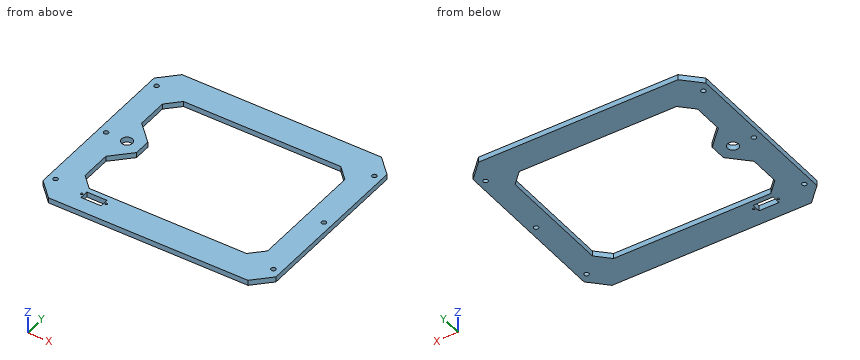
from build123d import *

# Parameters (mm, degrees)
SKETCH1_W           = 278
SKETCH1_H           = 238
BOSS_EXTRUDE1_DEPTH = 6.35
CHAMFER1_SIZE       = 20
SKETCH4_R           = 2.75
CUT_EXTRUDE2_DEPTH  = 76.2
SKETCH5_R           = 6.5
CUT_EXTRUDE3_DEPTH  = 10
SKETCH7_R           = 1.25
SKETCH7_W           = 24
SKETCH7_H           = 10.5
CUT_EXTRUDE4_DEPTH  = 7.35


with BuildPart() as part:
    # Sketch1 → Boss-Extrude1 (new body)
    with BuildSketch(Plane.XY):
        Rectangle(SKETCH1_W, SKETCH1_H)
    extrude(amount=BOSS_EXTRUDE1_DEPTH)

    # Chamfer1
    chamfer1_edges = [part.edges().sort_by_distance(p)[0] for p in [
        (-139, 119, 3.175),
        (139, 119, 3.175),
        (139, -119, 3.175),
        (-139, -119, 3.175),
    ]]
    chamfer(chamfer1_edges, length=CHAMFER1_SIZE)

    # Sketch4 → Cut-Extrude2 (cut)
    with BuildSketch(Plane.XY.offset(6.35)):
        with Locations((-130, 90)):
            Circle(SKETCH4_R)
        with Locations((-130, -90)):
            Circle(SKETCH4_R)
        with Locations((-130, 0)):
            Circle(SKETCH4_R)
        with Locations((130, -90)):
            Circle(SKETCH4_R)
        with Locations((130, 0)):
            Circle(SKETCH4_R)
        with Locations((130, 90)):
            Circle(SKETCH4_R)
    extrude(amount=-CUT_EXTRUDE2_DEPTH, mode=Mode.SUBTRACT)

    # Sketch5 → Cut-Extrude3 (cut)
    with BuildSketch(Plane.XY.offset(6.35)):
        with Locations((-105, 0)):
            Circle(SKETCH5_R)
        Polygon((93.875716073, -84), (-93.875716073, -84), (-108.875716073, -69), (-108.875716073, -32), (-86.875716073, -10), (-86.875716073, 10), (-108.875716073, 32), (-108.875716073, 69), (-93.875716073, 84), (93.875716073, 84), (108.875716073, 69), (108.875716073, -69), align=None)
    extrude(amount=-CUT_EXTRUDE3_DEPTH, mode=Mode.SUBTRACT)

    # Sketch7 → Cut-Extrude4 (cut, through all)
    with BuildSketch(Plane.XY.offset(6.35)):
        with Locations((-66.115841415, -95.342057099)):
            Circle(SKETCH7_R)
        with Locations((-95.115841415, -95.342057099)):
            Circle(SKETCH7_R)
        with Locations((-80.615841415, -95.342057099)):
            Rectangle(SKETCH7_W, SKETCH7_H)
    extrude(amount=-CUT_EXTRUDE4_DEPTH, mode=Mode.SUBTRACT)


solid = part.part
Can you work these out from the model? Positions are in its coordinate system, mm. Round coordinates to 2 decimals unless told otherwise and drop trailing zeros. Write each loop counter-clockwise with the first axis right and the second up, starting at its lowest first coordinate (ties: lowest second). Pieces come first, ordered by that corner, then holes. Notation, with made-up numbers: M -39,-27 L 10,-27 A25 ccw 10,-13 Z; hole C 39,62.25 d7. An arc over 180 degrees is marked long. Use CSV: the item, a comma, the result in double quotes.
(1) Imagine slicing it at A-A (x = 24). Write out the boundary of the cut face in (y, z), plus the area to 4 significant figures.
Check values:
outline,"M -119,0 L -84,0 L -84,6.35 L -119,6.35 Z; M 84,0 L 119,0 L 119,6.35 L 84,6.35 Z"
area,"444.5 mm^2"
(2) Imagine slicing it at B-B (y = -48). Write out the boundary of the cut face in (x, z).
Check values:
outline,"M -139,0 L -108.88,0 L -108.88,6.35 L -139,6.35 Z; M 108.88,0 L 139,0 L 139,6.35 L 108.88,6.35 Z"
(3) Imagine slicing it at C-C (z = 1.5). Count the separate pieces of the cut face and the enclosed holes in it, plus the area to 3 significant figures.
Check values:
separate pieces,"1"
enclosed holes,"11"
area,"29,600 mm^2"
(4) I need wall thicknesses on line 1 along Y through (x, z) = (-83, 5.25); line 2 along Y through (x, z) = (37, 2.75); line 3 along Y through (x, z) = (-105, 3). Which ranges of each line are inside material? Lowest first, please.
Check values:
line 1,"-119 to -100.59, -90.09 to -84, 84 to 119"
line 2,"-119 to -84, 84 to 119"
line 3,"-119 to -72.88, -28.12 to -6.5, 6.5 to 28.12, 72.88 to 119"
(5) Imagine slicing it at D-D (x = -105). Write out the boundary of the cut face in (y, z), plus the area to 3 significant figures.
Check values:
outline,"M -119,0 L -72.88,0 L -72.88,6.35 L -119,6.35 Z; M -28.12,0 L -6.5,0 L -6.5,6.35 L -28.12,6.35 Z; M 6.5,0 L 28.12,0 L 28.12,6.35 L 6.5,6.35 Z; M 72.88,0 L 119,0 L 119,6.35 L 72.88,6.35 Z"
area,"860 mm^2"
